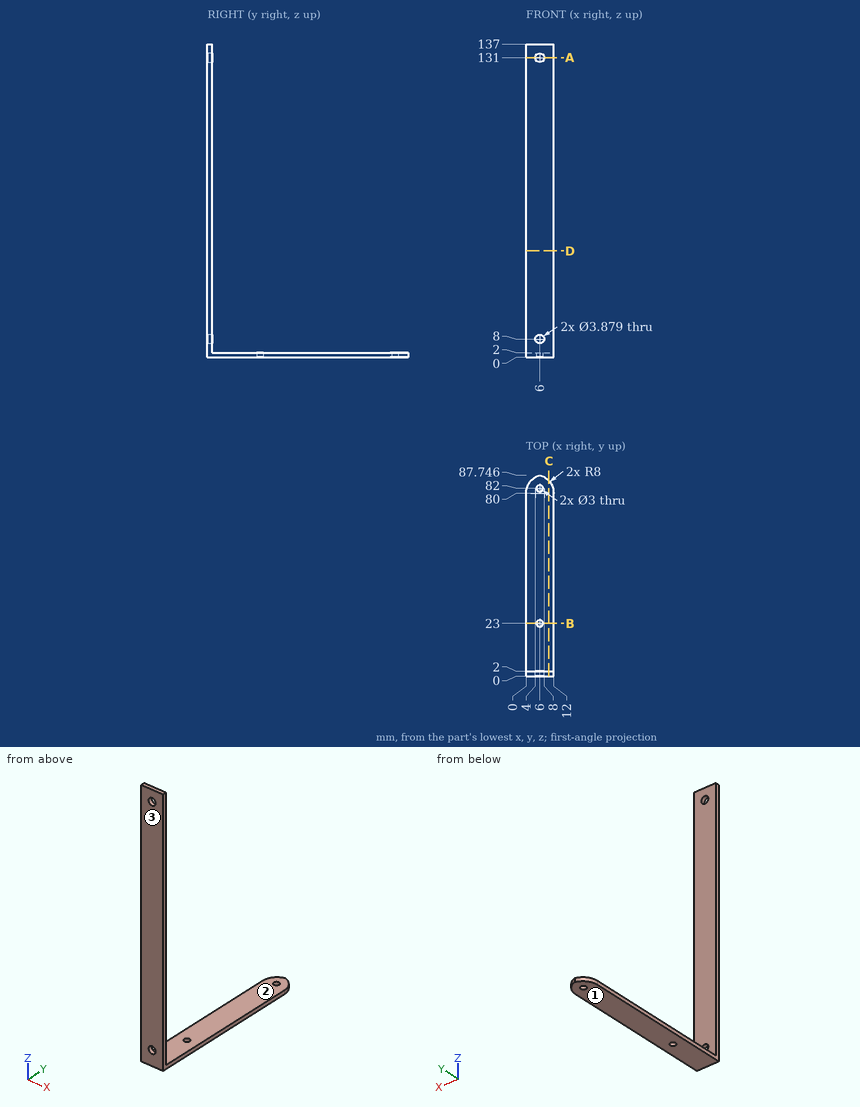
Input: dimensioned drawing with shaded views. Units: mm. Origin: part minimum x, y, z. Coordinates: 2 decimals unless noted, no trailing zeros. Write each loop counter-clockwise with the first axis right and the second up, starting at its lowest first coordinate (ties: lowest second). Pieces come first, ordered by that corner, then holes. Notation, with made-up numbers: M 18.25,25.25 L 40.25,25.25 A14 cw 40.25,44.25 Z; hole C 26.25,23 d11. An arc over 180 degrees is marked long. Use a Markdown table: item, result.
1) Mould query, pull axis Z, two halves, no side actions, for the marked faces 1, 2 and 3. Classes: pulls with the +Z half, pulls with the -Z half, needs draft (parallel to the pull), parting line crosses it, or undercut.
Conclusion:
| item | result |
|---|---|
| face 1 | pulls with the -Z half |
| face 2 | pulls with the +Z half |
| face 3 | needs draft |
2) First-contact query: pin 1 Ø2 at (x, z) = (6.5, 107) entering from -Y; pin 2 Ø4 at (x, z) = (1.5, 26) entering from +Y; pin 3 Ø5 at (x, y) = (6, 23) entering from +Z. Flat tips, straight axial feed; report the tip coordinate or a pass-through.
Conclusion:
| item | result |
|---|---|
| pin 1 | stops at y = 0 |
| pin 2 | stops at y = 2 |
| pin 3 | stops at z = 2 |
3) Section A-A, the plane z = 131. Output: boundary loops of the cut face in (x, y).
Conclusion:
| item | result |
|---|---|
| outline | M 0,0 L 4.06,0 L 4.06,2 L 0,2 Z; M 7.94,0 L 12,0 L 12,2 L 7.94,2 Z |
4) Section C-C, the plane x = 10. Output: boundary loops of the cut face in (y, z).
Conclusion:
| item | result |
|---|---|
| outline | M 0,0 L 85.29,0 L 85.29,2 L 2,2 L 2,137 L 0,137 Z |
5) Ray query, L1, parallel to Y at x = 6, z = 0.95; L2, parallel to X at y = 0.95, z = 8; L3, parallel to Y at x = 8, z = 100.5. Return the intervals inside material, ascending.
Conclusion:
| item | result |
|---|---|
| L1 | y = 0 to 21.5, 24.5 to 80.5, 83.5 to 87.75 |
| L2 | x = 0 to 4.06, 7.94 to 12 |
| L3 | y = 0 to 2 |
6) Section B-B, the plane y = 23. Output: boundary loops of the cut face in (x, z).
Conclusion:
| item | result |
|---|---|
| outline | M 0,0 L 4.5,0 L 4.5,2 L 0,2 Z; M 7.5,0 L 12,0 L 12,2 L 7.5,2 Z |
7) Section D-D, the plane z = 46.5. Output: boundary loops of the cut face in (x, y).
Conclusion:
| item | result |
|---|---|
| outline | M 0,0 L 12,0 L 12,2 L 0,2 Z |
